Here's the drawing with two shaded views (mm, measured from the low corner). I have some questions. A direction names the side the tool comes from. Coordinates: 2 decimals unless noted, no trailing zeros. Write each loop counter-clockwise with the first axis right and the second up, starting at its lowest first coordinate (ties: lowest second). Pieces come first, ordered by that corner, then holes. Notation, with made-up numbers: (43.25, 58) -> (52.25, 58) arc R16 cw to (52.25, 75) -> close; hole circle Ø7 at (86.5, 10.5). An arc over 180 degrees is marked (long way). Use a Markdown table: item, result. Add a question column.
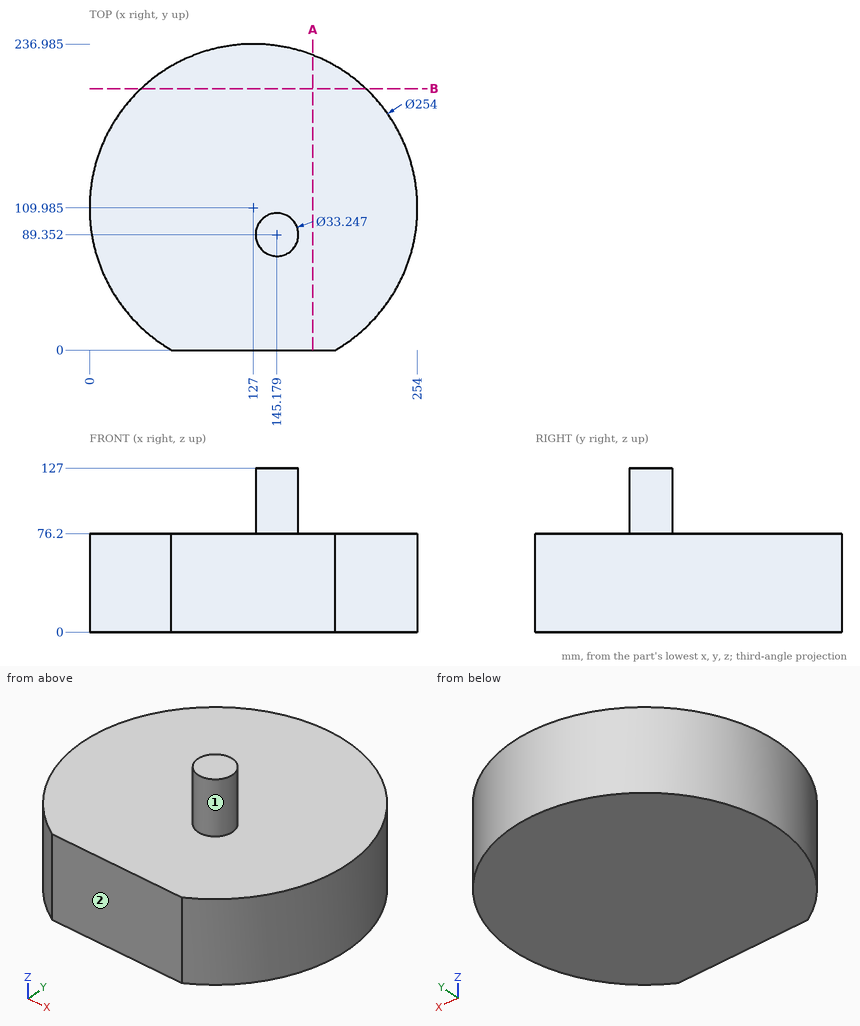
Q1. Suppose I cut it at A-A, the plane x = 173. Write out the boundary of the cut face in (y, z), and give its area (3 significant figures).
Q2. Suppose I cut it at B-B, the plane y = 202.5. Write out the boundary of the cut face in (x, z), and give its area (3 significant figures).
Q3. Which directions (+Z, -Z, +X, -X, +Y, -Y) give clear straight access to the entire face, cutting with the end or side of a thin tool? Please do the marked faces 1 and 2.
Q4. Will these pins go through, and if not, where does the flat tip stop? pin 1 (5 mm diameter, centred on x = 188.5, z = 67, fed in from +Y); pin 2 (1.5 mm diameter, centred on x = 141.5, z = 79, fed in from +Y); pin 3 (8 mm diameter, centred on x = 72, y = 29.5, fed in from +Z).
Q5. Please list where these lines run through material, in increasing order: line 1 (Z direction, x = 215.5, y = 88); line 2 (Y direction, x = 125.5, z = 15.5); line 3 (Y direction, x = 99.5, z = 57).
Answer key:
| question | item | result |
|---|---|---|
| 1 | outline | (0, 0) -> (228.36, 0) -> (228.36, 76.2) -> (0, 76.2) -> close |
| 1 | area | 17,400 mm^2 |
| 2 | outline | (39.99, 0) -> (214.01, 0) -> (214.01, 76.2) -> (39.99, 76.2) -> close |
| 2 | area | 13,300 mm^2 |
| 3 | face 1 | +Z |
| 3 | face 2 | +Z, -Z, +X, -X, -Y |
| 4 | pin 1 | stops at y = 222.45 |
| 4 | pin 2 | stops at y = 105.72 |
| 4 | pin 3 | stops at z = 76.2 |
| 5 | line 1 | z = 0 to 76.2 |
| 5 | line 2 | y = 0 to 236.98 |
| 5 | line 3 | y = 0 to 233.97 |
